For this review, use the dimensioned drawing (mm, ordinates from the lowest corner) and the shaded views. Coordinates: 2 decimals unless noted, no trailing zeros. Loops run counter-clockwise (first coordinate to the right, second up) from the corner with the lowest first, then second, coordinate; pieces in that order, holes last. Notation, with made-up numbers: M 35.5,27 L 80.5,27 A19 cw 80.5,46 Z; hole C 21.25,-40 d11. An arc over 180 degrees is marked long. Write item = value, one per line. Start each with the question number.
Q1. Clearance check with a flat-ended pin moving along its axis: pin 1 Ø1 at (x, y) = (13, 2) entering from -Z. State where the tip first meets the part, or that it passes through.
Q2. We need section B-B on z = 3. Give the boundary of the cut face in (x, y).
Q3. We need section C-C on y = 1.25. Count the separate pieces of the cut face and the enclosed holes in it, and give its area (3 significant figures).
Q4. Wall thickness on probe 1 along Z at (x, y) = (25.5, 0.8); probe 2 along X at (y, z) = (0.15, 36); probe 3 along Z at (x, y) = (35.5, 1): over which ranges is each line inside the solid? List them lowest first.
Q5. We need section D-D on x = 48. Give the boundary of the cut face in (y, z).
Q6. We need section A-A on x = 25.5. Give the boundary of the cut face in (y, z), and give its area (3 significant figures).
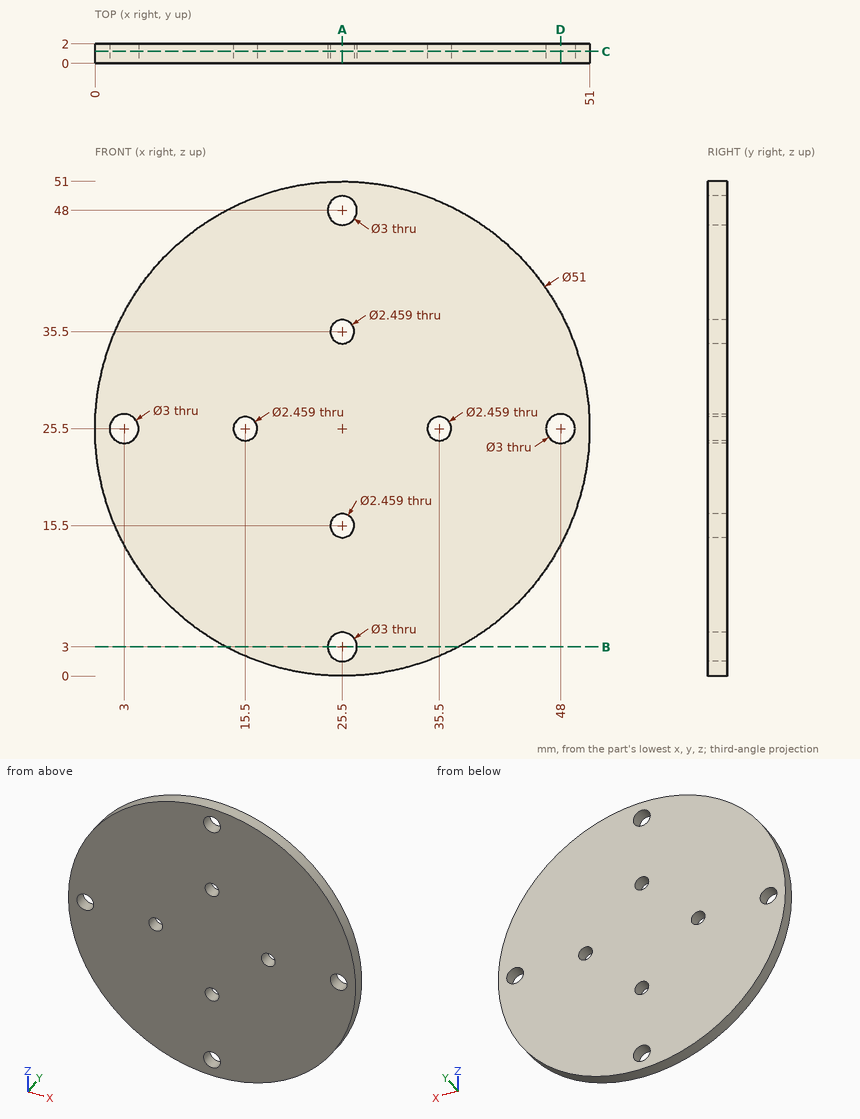
Returned:
q1.pin_1 = 3
q2.outline = M 13.5,0 L 24,0 L 24,2 L 13.5,2 Z; M 27,0 L 37.5,0 L 37.5,2 L 27,2 Z
q3.separate_pieces = 1
q3.enclosed_holes = 8
q3.area = 2,000 mm^2
q4.probe_1 = 0 to 1.5, 4.5 to 14.27, 16.73 to 34.27, 36.73 to 46.5, 49.5 to 51
q4.probe_2 = 2.26 to 24.38, 26.62 to 48.74
q4.probe_3 = 2.04 to 24.27, 26.73 to 48.96
q5.outline = M 0,13.5 L 2,13.5 L 2,24 L 0,24 Z; M 0,27 L 2,27 L 2,37.5 L 0,37.5 Z
q6.outline = M 0,0 L 2,0 L 2,1.5 L 0,1.5 Z; M 0,4.5 L 2,4.5 L 2,14.27 L 0,14.27 Z; M 0,16.73 L 2,16.73 L 2,34.27 L 0,34.27 Z; M 0,36.73 L 2,36.73 L 2,46.5 L 0,46.5 Z; M 0,49.5 L 2,49.5 L 2,51 L 0,51 Z
q6.area = 80.2 mm^2
